Autodesk Inventor part; units mm, degrees
ref_plane "YZ Plane" through (0, 0, 0) normal (1, 0, 0) x (0, 1, 0)
ref_plane "XZ Plane" through (0, 0, 0) normal (0, 1, 0) x (-1, 0, 0)
ref_plane "XY Plane" through (0, 0, 0) normal (0, 0, 1) x (1, 0, 0)
sketch "Boceto1" plane through (0, 0, 0) normal (0, 0, 1) x (1, 0, 0)
  line L0 (-32, -32) -> (32, -32)
  line L1 (32, -32) -> (32, 32)
  line L2 (32, 32) -> (-32, 32)
  line L3 (-32, 32) -> (-32, -32)
  line L4 (-32, -32) -> (32, 32) construction
  line L5 (32, -32) -> (-32, 32) construction
  point P0 (0, 0)
  dimension "d0" = 64
  dimension "d1" = 64
extrude "Extrusión1" add sketch "Boceto1" along normal blind 3
sketch "Boceto2" plane through (32, -32, 0) normal (1, 0, 0) x (0, 0, -1)
  line L0 (-74, 16.5) -> (1, 16.5)
  arc A0 (1, 10.5) -> (1, 16.5) centre (1, 13.5) ccw
  line L1 (1, 10.5) -> (-74, 10.5)
  line L2 (-74, -4.5) -> (-74, 10.5)
  line L3 (7, -4.5) -> (-74, -4.5)
  line L4 (7, -4.5) -> (7, 68.5)
  line L5 (7, 68.5) -> (-74, 68.5)
  line L6 (-74, 53.5) -> (-74, 68.5)
  line L7 (-74, 53.5) -> (1, 53.5)
  arc A1 (1, 47.5) -> (1, 53.5) centre (1, 50.5) ccw
  line L8 (1, 47.5) -> (-74, 47.5)
  line L9 (-74, 16.5) -> (-74, 47.5)
  line L10 (0, 0) -> (0, 64)
  line L11 (0, 64) -> (-3, 64)
  line L12 (-3, 0) -> (-3, 64)
  line L13 (0, 0) -> (-3, 0)
  line L14 (0, 47.5) -> (-3, 47.5)
  line L15 (-3, 47.5) -> (-3, 53.5)
  line L16 (-3, 53.5) -> (0, 53.5)
  line L17 (0, 53.5) -> (0, 47.5)
  line L18 (0, 47.7) -> (-3, 47.7)
  line L19 (-2.8, 47.7) -> (-2.8, 53.3)
  line L20 (-3, 53.3) -> (0, 53.3)
  line L21 (-0.2, 53.3) -> (-0.2, 47.7)
  point P0 (0, 32)
  dimension "d4" = 0.2
extrude "Extrusión2" add sketch "Boceto2" along normal blind 10 contours L12 L20 L19 L18 | L18 L21 L20 L10 | L19 L20 L21 L18
sketch "Boceto3" plane through (42, -32, 0) normal (1, 0, 0) x (0, 0, -1)
  line L0 (-3, 53.3) -> (-3, 47.7)
  line L1 (-3, 47.7) -> (0, 47.7)
  line L2 (0, 47.7) -> (0, 53.3)
  line L3 (0, 53.3) -> (-3, 53.3)
  line L4 (0, 47.7) -> (-3, 53.3)
  circle A0 centre (-1.5, 50.5) radius 5
  line L5 (-3, 53.3) -> (-3, 55.2697)
  line L6 (-3, 47.7) -> (0, 47.7)
  line L7 (0, 47.7) -> (0, 53.3)
  line L8 (0, 53.3) -> (-3, 53.3)
  line L9 (-3, 53.3) -> (-3, 47.7)
  line L10 (-3, 47.7) -> (-3, 42)
  point P0 (0, 32)
  point P1 (-3, 45.7303)
  dimension "d7" = 10
extrude "Extrusión3" add sketch "Boceto3" along normal blind 3 contours L4 L1 L0 | L5 A0 L10 L1 L2 L3 | L3 L2 L4
ref_plane "Plano de trabajo1" through (0, -32, 3) normal (1, 0, 0) x (0, 0, -1)
ref_plane "Plano de trabajo2" through (-32, 0, 0) normal (0, 1, 0) x (1, 0, 0)
mirror "Simetría1" about plane through (-32, 0, 0) normal (0, 1, 0) of "Extrusión2", "Extrusión3"
mirror "Simetría2" about plane through (0, -32, 3) normal (1, 0, 0) of "Extrusión2", "Simetría1", "Extrusión3"
properties part number "Parte deslizante"
Input: part model. Units: mm. Frame: model coordinates. A direction names the side the tool comes from. Give positions to 0.01 mm unless a question says otherwise; leave off trailing zeros. Write each loop counter-clockwise with the first axis right and the second up, starting at its lowest first coordinate (ties: lowest second). Pieces come first, ordered by that corner, then holes.
Q1. Section B-B, the plane y = 18.5. Output: boundary loops of the cut face in (x, z), plus the area to 3 significant figures.
Q2. Pull-direction query (Y, two-part tool) for faces 4 (the face through (-43.5, -18.6, -3.5)), 5 (the face through (-37, -21.3, 2)), 6 (the face through (-1, 0, 0)); classes: pulls with the +Y half, pulls with the -Y half, needs draft (parallel to the pull), parting line crosses it, or undercut.
Q3. First-contact query: P1, Ø2, axis at y = 4.5, z = 1.5, coming from the -X side; P2, Ø2, axis at y = 0.5, z = -2.5, coming from the +X side (3 decimals); P3, Ø2.5, axis at x = 39, z = 1, coming from the -Y side; P4, Ø3.5, axis at y = 28.5, z = 1.5, coming from the +X side. Flat tips, straight axial feed; report the tip coordinate or a pass-through.
Q4. Set-up query: faces 1 (the face through (42, -18.6, -0.3)), 2 (the face through (32, 0, 1)), 3 (the face through (32, 27, 1)). Return all of +Z, -Z, +X, -X, +Y, -Y with unobstructed straight access to the full face (end or side cutting, diameter ignored); none if empty.
Q5. Section A-A, the plane x = -33. Output: boundary loops of the cut face in (y, z).
Q6. Section D-D, the plane y = 3. Output: boundary loops of the cut face in (x, z).
Q7. Section C-C, the plane z = -2. Output: boundary loops of the cut face in (x, y).
Q8. Material intervals for probe 1 along X at (y, z) = (-17.5, -0.75); probe 2 along X at (y, z) = (21.5, 0.75); probe 3 along Y at (x, z) = (37, 1.5), sorted ascending.
Filled in:
1. outline: (-45, -3.5) - (-42, -3.5) - (-42, 0) - (42, 0) - (42, -3.5) - (45, -3.5) - (45, 3) - (-45, 3) - close
1. area: 291 mm2
2. face 4: undercut
2. face 5: pulls with the -Y half
2. face 6: needs draft
3. P1: stops at x = -32
3. P2: passes through
3. P3: stops at y = -21.3
3. P4: stops at x = 32
4. face 1: -Z
4. face 2: +Z, -Z
4. face 3: +Z, -Z, +Y
5. outline: (-21.3, 0) - (-15.7, 0) - (-15.7, 3) - (-21.3, 3) - close; (15.7, 0) - (21.3, 0) - (21.3, 3) - (15.7, 3) - close
6. outline: (-32, 0) - (32, 0) - (32, 3) - (-32, 3) - close
7. outline: (-45, -22.07) - (-42, -22.07) - (-42, -14.93) - (-45, -14.93) - close; (-45, 14.93) - (-42, 14.93) - (-42, 22.07) - (-45, 22.07) - close; (42, -22.07) - (45, -22.07) - (45, -14.93) - (42, -14.93) - close; (42, 14.93) - (45, 14.93) - (45, 22.07) - (42, 22.07) - close
8. probe 1: x = -45 to -42, 42 to 45
8. probe 2: x = -45 to -42, -32 to 32, 42 to 45
8. probe 3: y = -21.3 to -15.7, 15.7 to 21.3
